Work out the finished part from the listing and answer in its coordinate system (mm). Face numbers are marked on the shaded views. A direction names the side the tool comes from. Coordinates: 2 decimals unless noted, no trailing zeros. Answer as a JSON object with one key per item and string values. Group by question number.
1) The mould has two halves that part along Y. Classify the marked faces 4, 5 and 6: released by +Y, released by -Y, zero draft, split by the parting line, or undercut.
2) Find the intervals of material crossed by line 1 along Z through (x, y) = (6.85, 0); line 2 along Y through (x, z) = (7.1, 0); line 3 along Z through (x, y) = (-4.5, 9), in increasing order.
3) Each of these flat-tipped pins is pushed along its axis until it touches: P1, Ø2, axis at y = -3, z = 28, coming from the +X side; P2, Ø5, axis at x = -5.5, y = -10, coming from the +Z side; P3, Ø20, axis at y = -2, z = -8.5, coming from the -X side. Where does it stop, or does it pass through?
4) A tool of negligible diameter and unlimited length cuts with its end or side. For the marked faces 1, 2 and 3, from which of +Z, -Z, +X, -X, +Y, -Y can it reach the whole face along a straight path? Write none if from no direction.
Solid Edge part; units mm, degrees
sketch "Sketch1" plane through (0, 0, 0) normal (0, -1, 0) x (1, 0, 0)
  line L0 (-8, 17.5) -> (-8, 62)
  line L1 (-8, 62) -> (-6, 62)
  line L2 (-6, 62) -> (-1.7877, 53.6032)
  arc A0 (-1.7877, 53.6032) -> (0, 52.5) centre (0, 54.5) ccw
  line L3 (0, 52.5) -> (0, 17.5)
  line L4 (0, 17.5) -> (-8, 17.5)
revolve "RevolvedProtrusion1" add sketch "Sketch1" angle 360 about axis through (-60, 0, 0) along (1, 0, 0)
mirror "Mirror1" about plane through (0, 0, 0) normal (1, 0, 0) of "RevolvedProtrusion1"
sketch "Sketch2" plane through (-8, 0, 0) normal (-1, 0, 0) x (0, -1, 0)
  circle A0 centre (0, 0) radius 20
extrude "Cutout1" cut sketch "Sketch2" against normal blind 14
chamfer "Fase_1" distance 1 angle 45 1 edges at (-8, 20, 0)
sketch "Sketch3" plane through (0, 0, 0) normal (0, 0, 1) x (1, 0, 0)
  line L0 (8, 57) -> (8, 25)
  line L1 (8, 25) -> (5, 25)
  arc A0 (5, 25) -> (3, 27) centre (5, 27) cw
  line L2 (3, 27) -> (3, 44.6654)
  arc A1 (3, 44.6654) -> (4.0617, 49.1494) centre (13, 44.6654) cw
  line L3 (4.0617, 49.1494) -> (8, 57)
revolve "RevolvedCutout1" cut sketch "Sketch3" angle 360 about axis through (57, 0, 0) along (-1, 0, 0)
mirror "Mirror2" about plane through (0, 0, 0) normal (1, 0, 0) of "RevolvedCutout1"
properties material "Aluminium, 1060"
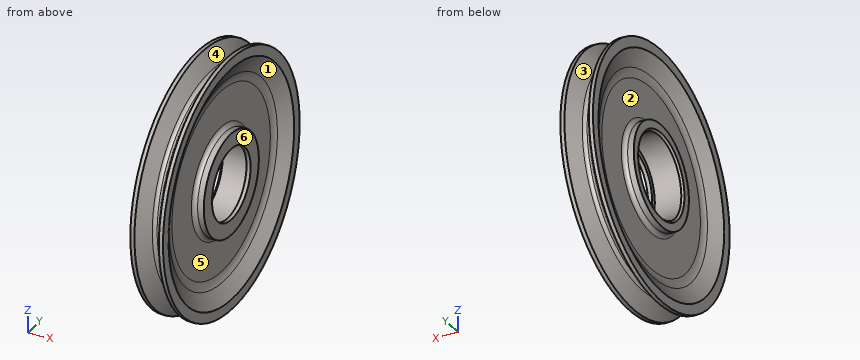
Report:
{
 "1": {"face 4": "split by the parting line", "face 5": "undercut", "face 6": "zero draft"},
 "2": {"line 1": "z = -62 to -54.71, -25 to -17.5, 17.5 to 25, 54.71 to 62", "line 2": "y = -62 to -55.21, -25 to -17.5, 17.5 to 25, 55.21 to 62", "line 3": "z = -58.32 to -49.21, -23.39 to -17.86, 17.86 to 23.39, 49.21 to 58.32"},
 "3": {"P1": "stops at x = 3", "P2": "stops at z = 61.54", "P3": "stops at x = 6"},
 "4": {"face 1": "+X", "face 2": "-X", "face 3": "none"}
}
